Design review of the part shown in the three views and the two pictorial views. Dimensions are in mm from the part's minimum x, y and z. A direction names the side the tool comes from. Coordinates: 2 decimals unless noted, no trailing zeros. Write each loop counter-clockwise with the first axis right and the second up, starting at its lowest first coordinate (ties: lowest second). Pieces come first, ordered by that corner, then holes.
Q1. For pin 1 Ø1.5 at (x, y) = (9.5, 22) entering from +Z (3 decimals); pin 2 Ø2 at (x, z) = (20, 7) entering from +Y (3 decimals), all flat-tipped, find the tip position at first contact; note any pin that passes through.
Q2. For L1, parallel to X at y = 2.25, z = 38.1 (3 decimals); L2, parallel to X at y = 2.25, z = 13.5; L3, parallel to Z at x = 19.5, y = 6.75 (3 decimals), list the stretches that pass through material, from the lowest coordinate up.
Q3. Take a section at D-D, the plane x = 47. Write out the cut boundary in (y, z) (3 decimals).
Q4. Take a section at A-A, the plane y = 12.7. Write out the cut boundary in (x, z) (3 decimals).
Q5. For the marked faces 1 and 2, list the 3-axis set-ups (+Z, -Z, +X, -X, +Y, -Y) from which the entire face can be reached by the end or side of a thin tool; tool diameter is ignored.
Q6. Take a section at C-C, the plane x = 38.1. Write out the cut boundary in (y, z) (3 decimals).
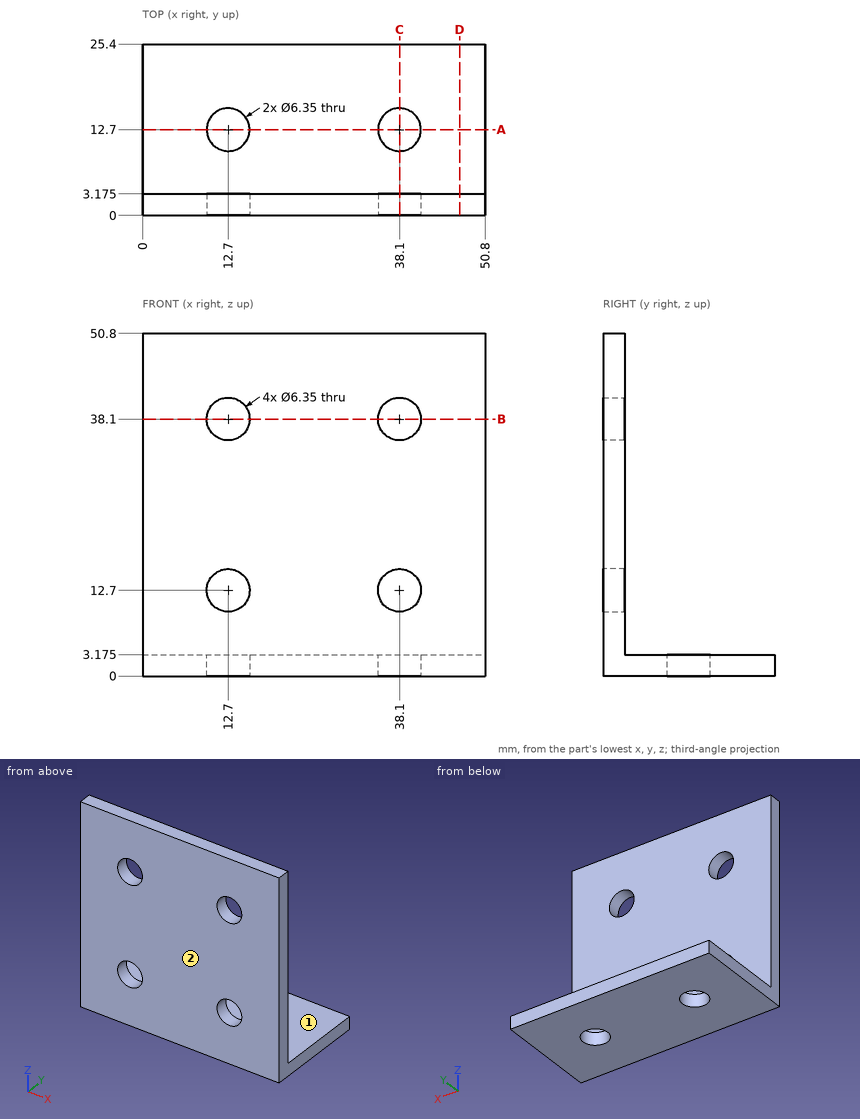
Responses:
1. pin 1: stops at z = 3.175
1. pin 2: stops at y = 3.175
2. L1: x = 0 to 9.525, 15.875 to 34.925, 41.275 to 50.8
2. L2: x = 0 to 9.63, 15.77 to 35.03, 41.17 to 50.8
2. L3: z = 0 to 3.175
3. outline: (0, 0) - (25.4, 0) - (25.4, 3.175) - (3.175, 3.175) - (3.175, 50.8) - (0, 50.8) - close
4. outline: (0, 0) - (9.525, 0) - (9.525, 3.175) - (0, 3.175) - close; (15.875, 0) - (34.925, 0) - (34.925, 3.175) - (15.875, 3.175) - close; (41.275, 0) - (50.8, 0) - (50.8, 3.175) - (41.275, 3.175) - close
5. face 1: +Z, +X, -X, +Y
5. face 2: +Z, -Z, +X, -X, -Y
6. outline: (0, 0) - (9.525, 0) - (9.525, 3.175) - (3.175, 3.175) - (3.175, 9.525) - (0, 9.525) - close; (0, 15.875) - (3.175, 15.875) - (3.175, 34.925) - (0, 34.925) - close; (0, 41.275) - (3.175, 41.275) - (3.175, 50.8) - (0, 50.8) - close; (15.875, 0) - (25.4, 0) - (25.4, 3.175) - (15.875, 3.175) - close
